Geometry: see drawing. Coordinates: mm, zero at the bounding-box minimum. Coordinates: 2 decimals unless noted, no trailing zeros. Order: outer loops, then holes, each group sorted by start corner. A loop starts at its lowest first (then second) coordinate and runs counter-clockwise, first axis right, second up.
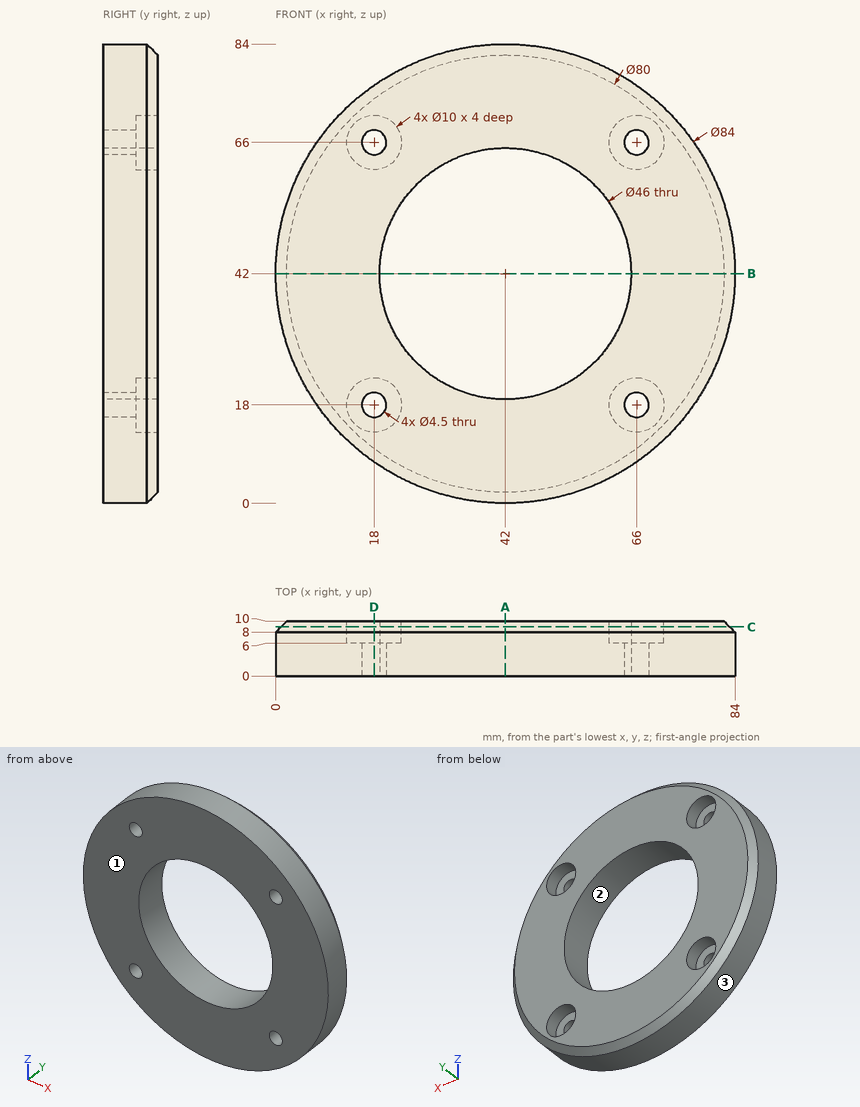
Q1. Section query D-D on x = 18. Give the number of separate pieces and of enclosed holes in the cut face, plus the area to 3 significant figures.
Solutions:
separate pieces: 3
enclosed holes: 0
area: 550 mm2
Q2. Section query A-A on x = 42. Output: boundary loops of the cut face in (y, z), plus the area to 3 significant figures.
Solutions:
outline: (0, 0) - (8, 0) - (10, 2) - (10, 19) - (0, 19) - close; (0, 65) - (10, 65) - (10, 82) - (8, 84) - (0, 84) - close
area: 376 mm2
Q3. Pin query (flat end, axial travel): P1, Ø6, axis at x = 66, z = 66, coming from the +Y side; P2, Ø3, axis at x = 11, y = 8.5, coming from the -Z side; P3, Ø3, axis at y = 4, z = 56.5, coming from the -X side; P4, Ø3, axis at x = 65.5, z = 18, coming from the +Y side. Return the tip coordinate at first contact, or that it passes through.
Solutions:
P1: stops at y = 6
P2: stops at z = 12.19
P3: stops at x = 2.06
P4: passes through
Q4. Pull-direction query (Z, two-part tool) for the marked faces 1, 2 and 3; classes: pulls with the +Z half, pulls with the -Z half, needs draft (parallel to the pull), parting line crosses it, or undercut.
Solutions:
face 1: needs draft
face 2: undercut
face 3: parting line crosses it
Q5. Material intervals for line 1 along X through (y, z) = (4.45, 18); line 2 along X through (y, z) = (3.5, 42); line 3 along X through (y, z) = (8.65, 66), sorted ascending.
Solutions:
line 1: x = 7.53 to 15.75, 20.25 to 63.75, 68.25 to 76.47
line 2: x = 0 to 19, 65 to 84
line 3: x = 8.33 to 13, 23 to 61, 71 to 75.67
Q6. Section query B-B on z = 42. Output: boundary loops of the cut face in (x, y), plus the area to 3 significant figures.
Solutions:
outline: (0, 0) - (19, 0) - (19, 10) - (2, 10) - (0, 8) - close; (65, 0) - (84, 0) - (84, 8) - (82, 10) - (65, 10) - close
area: 376 mm2
Q7. Section query C-C on y = 9. Output: boundary loops of the cut face in (x, z), plus the area to 3 significant figures.
Solutions:
outline: circle Ø82 at (42, 42); hole circle Ø10 at (18, 18); hole circle Ø10 at (18, 66); hole circle Ø46 at (42, 42); hole circle Ø10 at (66, 18); hole circle Ø10 at (66, 66)
area: 3,300 mm2
